from build123d import *

# Parameters (mm, degrees)
SKETCH_1_R             = 8
SM_BASE_FLANGE_1_DEPTH = 4
CHAMFER_1_SIZE         = 2


# Sheet-metal steps are written as plain solids
with BuildPart() as part:
    # Sketch 1 → Базовая кромка1 (new body)
    with BuildSketch(Plane.XY):
        with BuildLine():
            Line((0, 16), (-65, 16))
            Line((-65, 16), (-65, -16))
            Line((-65, -16), (0, -16))
            ThreePointArc((0, -16), (16, 0), (0, 16))
        make_face()
        Circle(SKETCH_1_R, mode=Mode.SUBTRACT)
    extrude(amount=SM_BASE_FLANGE_1_DEPTH)

    # Фаска1
    chamfer_1_edges = [part.edges().sort_by_distance(p)[0] for p in [
        (-8, 0, 4),
    ]]
    chamfer(chamfer_1_edges, length=CHAMFER_1_SIZE)


solid = part.part
Read the model definition and answer for the solid it produces. Units are mm, in the model's axes. Coordinates: 2 decimals unless noted, no trailing zeros. Order: outer loops, then holes, each group sorted by start corner. A loop starts at its lowest first (then second) coordinate and runs counter-clockwise, first axis right, second up. Notation, with made-up numbers: M 27.25,76 L 54.25,76 A24 ccw 54.25,108 Z; hole C 26.5,16.25 d7. An arc over 180 degrees is marked long. Put each result on its own line as item: value. Start each with the question number.
Item 1: Consider probe 1 along X at (y, z) = (2.5, 0.25); probe 2 along X at (y, z) = (0.5, 3.2); probe 3 along Y at (x, z) = (9, 0.8). Determine where each line is inside the solid, lowest interval first. Write a range as [from, to].
Item 2: Section A-A, the plane y = 0 is taken. Determine the outline of the cut face in (x, z).
Item 3: Section B-B, the plane z = 3.4 is taken. Determine the outline of the cut face in (x, y), plus the area to 3 significant figures.
Item 4: Given pin 1 Ø18.5 at (x, y) = (0, 0) entering from +Z; pin 2 Ø1 at (y, z) = (7.5, 3.5) entering from +X, each flat-ended and moving along its own axis, determine where each tip first touches the part or whether it passes through.
Item 5: The mould has two halves that part along X. Classify faces 1 (the face through (16, 0, 2)), 2 (the face through (-1.761, -7.932, 2.125)), 3 (the face through (-33, -16, 2)): +X half, -X half, draft (parallel to the pull), parting line (faces both ways), or undercut.
Computed:
1. probe 1: x = [-65, -7.6], [7.6, 15.8]
1. probe 2: x = [-65, -9.19], [9.19, 15.99]
1. probe 3: y = [-13.23, 13.23]
2. outline: M -65,0 L -8,0 L -8,2 L -10,4 L -65,4 Z; M 8,0 L 16,0 L 16,4 L 10,4 L 8,2 Z
3. outline: M -65,-16 L 0,-16 A16 ccw 0,16 L -65,16 Z; hole C 0,0 d18.8
3. area: 2,200 mm2
4. pin 1: stops at z = 3.25
4. pin 2: stops at x = 14.39
5. face 1: +X half
5. face 2: undercut
5. face 3: draft
